Read the model definition and answer for the solid it produces. Units are mm, in the model's axes. A direction names the side the tool comes from. Coordinates: 2 decimals unless noted, no trailing zeros. Write each loop counter-clockwise with the first axis right and the second up, starting at its lowest first coordinate (ties: lowest second). Pieces come first, ordered by that corner, then holes.
(1) Section A-A on y = -54.5 is taken. Write down the section's boundary in (x, z).
(2) Section D-D on y = -43.5 is taken. Write down the section's boundary in (x, z).
(3) Given pin 1 (12 mm diameter, centred on x = 21, y = -20, fed in from +Z); pin 2 (5.5 mm diameter, centred on x = 51, z = 8, fed in from -Y); pin 3 (8 mm diameter, centred on x = 42.5, y = -18.5, fed in from +Z); pin 4 (6 mm diameter, centred on y = -52.5, z = 20.5, fed in from +X), each flat-ended and moving along its own axis, determine where each tip first touches the part or whether it passes through.
(4) Which of the six approach directions +Z, -Z, +X, -X, +Y, -Y give full straight-line access (tool end or side, diameter ignored) to faces 1 (the flat face through (23.376, -51, 7)), 2 (the flat face through (47, 0, 28)), 3 (the flat face through (36, -10, 42))?
(5) Section B-B on x = 6.5 is taken. Write down the section's boundary in (y, z), then the cut area to 4 significant figures.
(6) The mould has two halves that part along X. Classify faces 4 (the flat face through (73.463, -51, 7)), 5 (the flat face through (46.835, -29.094, 22.272)), 6 (the flat face through (95, -24, 11)): +X half, -X half, draft (parallel to the pull), parting line (faces both ways), or undercut.
(7) Section C-C on z = 11.5 is taken. Write down the section's boundary in (x, y).
(8) Find the intervals of material crossed by probe 1 along X at (y, z) = (-42, 5); probe 2 along Y at (x, z) = (63.5, 49); probe 3 along Y at (x, z) = (50, 10.5), in increasing order.
from build123d import *

# Parameters (mm, degrees)
F1_DEPTH = 95
F3_DEPTH = 25
F4_W     = 50.086444
F4_H     = 18.488904
F5_DEPTH = 56.001


with BuildPart() as f1:
    # F0 (on Right) → F1 (new body)
    with BuildSketch(Plane.YZ):
        Polygon((-60, 0), (0, 0), (0, 56), (-10, 56), (-10, 28), (-60, 13), align=None)
    extrude(amount=F1_DEPTH)

    # F2 (on face) → F3 (cut)
    with BuildSketch(Plane.XZ.offset(10)):
        Polygon((56, 56), (95, 28), (95, 56), align=None)
    extrude(amount=-F3_DEPTH, mode=Mode.SUBTRACT)

    # F4 (on face) → F5 (cut, through all)
    with BuildSketch(Plane(origin=(0, 0, 0), x_dir=(1, 0, 0), z_dir=(0, 0, -1))):
        with Locations((48.419592, 50.755548)):
            Rectangle(F4_W, F4_H)
    extrude(amount=-F5_DEPTH, mode=Mode.SUBTRACT)


solid = f1.part
Response:
1. outline: (0, 0) - (23.38, 0) - (23.38, 14.65) - (0, 14.65) - close; (73.46, 0) - (95, 0) - (95, 14.65) - (73.46, 14.65) - close
2. outline: (0, 0) - (23.38, 0) - (23.38, 17.95) - (0, 17.95) - close; (73.46, 0) - (95, 0) - (95, 17.95) - (73.46, 17.95) - close
3. pin 1: stops at z = 26.8
3. pin 2: stops at y = -41.51
3. pin 3: stops at z = 26.65
3. pin 4: passes through
4. face 1: +Z, -Z, -Y
4. face 2: +Z, -Z, +X, -X, +Y
4. face 3: +Z, +X, -X, -Y
5. outline: (-60, 0) - (0, 0) - (0, 56) - (-10, 56) - (-10, 28) - (-60, 13) - close
5. area: 1,585 mm2
6. face 4: undercut
6. face 5: draft
6. face 6: +X half
7. outline: (0, -60) - (23.38, -60) - (23.38, -41.51) - (73.46, -41.51) - (73.46, -60) - (95, -60) - (95, 0) - (0, 0) - close
8. probe 1: x = 0 to 23.38, 73.46 to 95
8. probe 2: y = -10 to 0
8. probe 3: y = -41.51 to 0
